```python
from build123d import *

# Parameters (mm, degrees)
F0_W     = 25.4
F0_H     = 25.4
F1_DEPTH = 2.54
F3_DEPTH = 1.27
F4_W     = 0.508
F4_H     = 1.016
F6_W     = 0.508
F6_H     = 1.016
F8_W     = 0.508
F8_H     = 1.016
F10_W    = 0.508
F10_H    = 1.016


with BuildPart() as f1:
    # F0 (on Front) → F1 (new body)
    with BuildSketch(Plane.XZ):
        Rectangle(F0_W, F0_H)
    extrude(amount=F1_DEPTH)

    # F2 (on face) → F3 (join)
    with BuildSketch(Plane(origin=(0, 0, 0), x_dir=(-1, 0, 0), z_dir=(0, 1, 0))):
        Polygon((-10.668, 10.668), (-10.668, 11.684), (-11.176, 11.684), (-11.684, 11.684), (-11.684, 10.668), align=None)
        Polygon((11.684, 10.668), (11.684, 11.684), (11.176, 11.684), (10.668, 11.684), (10.668, 10.668), align=None)
        Polygon((-10.668, -11.684), (-10.668, -10.668), (-11.684, -10.668), (-11.684, -11.684), (-11.176, -11.684), align=None)
        Polygon((11.684, -11.684), (11.684, -10.668), (10.668, -10.668), (10.668, -11.684), (11.176, -11.684), align=None)
    extrude(amount=F3_DEPTH)

    # F4 (on face) → F5 (revolve)
    with BuildSketch(Plane(origin=(0, 1.27, 0), x_dir=(-1, 0, 0), z_dir=(0, 1, 0))):
        with BuildLine():
            ThreePointArc((-11.176, 10.414), (-10.6371846327, 10.6371846327), (-10.414, 11.176))
            ThreePointArc((-10.414, 11.176), (-10.6371846327, 11.7148153673), (-11.176, 11.938))
            Line((-11.176, 11.938), (-11.176, 11.684))
            Line((-11.176, 11.684), (-10.668, 11.684))
            Line((-10.668, 11.684), (-10.668, 10.668))
            Line((-10.668, 10.668), (-11.176, 10.668))
            Line((-11.176, 10.668), (-11.176, 10.414))
        make_face()
        with Locations((-10.922, 11.176)):
            Rectangle(F4_W, F4_H)
        with Locations((-11.43, 11.176)):
            Rectangle(F4_W, F4_H)
    revolve(axis=Axis((11.176, 1.27, 11.176), (0, 0, -1)))

    # F6 (on face) → F7 (revolve)
    with BuildSketch(Plane(origin=(0, 1.27, 0), x_dir=(-1, 0, 0), z_dir=(0, 1, 0))):
        with BuildLine():
            ThreePointArc((11.176, 10.414), (11.7148153673, 10.6371846327), (11.938, 11.176))
            ThreePointArc((11.938, 11.176), (11.7148153673, 11.7148153673), (11.176, 11.938))
            Line((11.176, 11.938), (11.176, 11.684))
            Line((11.176, 11.684), (11.684, 11.684))
            Line((11.684, 11.684), (11.684, 10.668))
            Line((11.684, 10.668), (11.176, 10.668))
            Line((11.176, 10.668), (11.176, 10.414))
        make_face()
        with Locations((11.43, 11.176)):
            Rectangle(F6_W, F6_H)
        with Locations((10.922, 11.176)):
            Rectangle(F6_W, F6_H)
    revolve(axis=Axis((-11.176, 1.27, 11.176), (0, 0, -1)))

    # F8 (on face) → F9 (revolve)
    with BuildSketch(Plane(origin=(0, 1.27, 0), x_dir=(-1, 0, 0), z_dir=(0, 1, 0))):
        with BuildLine():
            ThreePointArc((11.176, -11.938), (11.7148153673, -11.7148153673), (11.938, -11.176))
            ThreePointArc((11.938, -11.176), (11.7148153673, -10.6371846327), (11.176, -10.414))
            Line((11.176, -10.414), (11.176, -10.668))
            Line((11.176, -10.668), (11.684, -10.668))
            Line((11.684, -10.668), (11.684, -11.684))
            Line((11.684, -11.684), (11.176, -11.684))
            Line((11.176, -11.684), (11.176, -11.938))
        make_face()
        with Locations((11.43, -11.176)):
            Rectangle(F8_W, F8_H)
        with Locations((10.922, -11.176)):
            Rectangle(F8_W, F8_H)
    revolve(axis=Axis((-11.176, 1.27, -11.176), (0, 0, -1)))

    # F10 (on face) → F11 (revolve)
    with BuildSketch(Plane(origin=(0, 1.27, 0), x_dir=(-1, 0, 0), z_dir=(0, 1, 0))):
        with BuildLine():
            Line((-11.176, -10.668), (-11.176, -10.3170624905))
            ThreePointArc((-11.176, -10.3170624905), (-12.0349375095, -11.176), (-11.176, -12.0349375095))
            Line((-11.176, -12.0349375095), (-11.176, -11.684))
            Line((-11.176, -11.684), (-11.684, -11.684))
            Line((-11.684, -11.684), (-11.684, -10.668))
            Line((-11.684, -10.668), (-11.176, -10.668))
        make_face()
        with Locations((-10.922, -11.176)):
            Rectangle(F10_W, F10_H)
        with Locations((-11.43, -11.176)):
            Rectangle(F10_W, F10_H)
    revolve(axis=Axis((11.176, 1.27, -11.176), (0, 0, -1)))


solid = f1.part
```
Verification items for the finished model (mm, model axes). A direction names the side the tool comes from. Round coordinates to 2 decimals unless told otherwise and drop trailing zeros. Order: outer loops, then holes, each group sorted by start corner. A loop starts at its lowest first (then second) coordinate and runs counter-clockwise, first axis right, second up. Notation, with made-up numbers: (-7.75, 15.25) - (45.25, 15.25) arc R29 ccw to (45.25, 54.25) - close; hole circle Ø6 at (71.5, 70.5). An arc over 180 degrees is marked (long way). Use CSV: the item, a comma, the result in double quotes. Start each with the question number.
1) Access from +Z, -Z, +X, -X, +Y, -Y to the whole of each face (thin tool, end or side, straight path). Record for faces 4 (the flat face through (12.7, -1, 0)), 5 (the cylindrical face through (-11.187, 1.778, -11.169)).
2) Thickness scan on L1, parallel to Z at x = 11.25, y = 1.3; L2, parallel to Z at x = -11, y = 0.3. Record the ranges inside material, lowest first.
3) Mould release check, pull along Z, two halves, no side actions. Record for faces 1 (the flat face through (-12.7, -1, 0)), 2 (the flat face through (-11.2, 0.4, 10.668)), 3 (the flat face through (0, -1, -12.7)): +Z half, -Z half, draft (parallel to the pull), parting line (faces both ways), or undercut.
4) Section check A-A, the plane x = 10. Record the cut outline in (y, z).
5) Section check B-B, the plane z = 2.25. Record the cut outline in (x, y), plus the area to 3 significant figures.
6) Go/stop test with flat-tipped pins: P1, Ø0.8, axis at y = 0.5, z = 11, coming from the -X side; P2, Ø0.8, axis at x = 11, y = 0.5, coming from the -Z side; P3, Ø0.8, axis at y = 0.5, z = 11.5, coming from the +X side. Record where each tip stops, or that it passes through.
Answers:
1,face 4,"+Z, -Z, +X, +Y, -Y"
1,face 5,"none"
2,L1,"z = -12.03 to -11.68, -10.67 to -10.32, 10.42 to 10.67, 11.68 to 11.93"
2,L2,"z = -11.68 to -10.67, 10.67 to 11.68"
3,face 1,"draft"
3,face 2,"undercut"
3,face 3,"-Z half"
4,outline,"(-2.54, -12.7) - (0, -12.7) - (0, 12.7) - (-2.54, 12.7) - close"
5,outline,"(-12.7, -2.54) - (12.7, -2.54) - (12.7, 0) - (-12.7, 0) - close"
5,area,"64.5 mm²"
6,P1,"stops at x = -11.83"
6,P2,"stops at z = -11.94"
6,P3,"stops at x = 11.8"
